```python
from build123d import *

# Parameters (mm, degrees)
SKETCH1_R      = 2.6035
EXTRUDE1_DEPTH = 25.4


with BuildPart() as part:
    # Sketch1 → Extrude1 (new body)
    with BuildSketch(Plane.XY):
        with BuildLine():
            Line((10.5918, 12.7), (10.5664, 12.7))
            ThreePointArc((10.5664, 12.7), (10.0584, 12.192), (9.5504, 12.7))
            Line((9.5504, 12.7), (6.3246, 12.7))
            ThreePointArc((6.3246, 12.7), (5.8166, 12.192), (5.3086, 12.7))
            Line((5.3086, 12.7), (4.3561, 12.7))
            ThreePointArc((4.3561, 12.7), (3.2512, 11.5951), (4.3561, 10.4902))
            Line((4.3561, 10.4902), (6.370083786, 10.4902))
            ThreePointArc((6.370083786, 10.4902), (7.348856743, 9.836204819), (7.119204175, 8.681663397))
            Line((7.119204175, 8.681663397), (3.88464389, 5.447103113))
            ThreePointArc((3.88464389, 5.447103113), (2.854599758, 4.758849627), (1.63957986, 4.517167143))
            Line((1.63957986, 4.517167143), (-1.63957986, 4.517167143))
            ThreePointArc((-1.63957986, 4.517167143), (-2.854599758, 4.758849627), (-3.88464389, 5.447103113))
            Line((-3.88464389, 5.447103113), (-7.119204175, 8.681663397))
            ThreePointArc((-7.119204175, 8.681663397), (-7.348856743, 9.836204819), (-6.370083786, 10.4902))
            Line((-6.370083786, 10.4902), (-4.3561, 10.4902))
            ThreePointArc((-4.3561, 10.4902), (-3.2512, 11.5951), (-4.3561, 12.7))
            Line((-4.3561, 12.7), (-5.3086, 12.7))
            ThreePointArc((-5.3086, 12.7), (-5.8166, 12.192), (-6.3246, 12.7))
            Line((-6.3246, 12.7), (-9.5504, 12.7))
            ThreePointArc((-9.5504, 12.7), (-10.0584, 12.192), (-10.5664, 12.7))
            Line((-10.5664, 12.7), (-10.5918, 12.7))
            ThreePointArc((-10.5918, 12.7), (-12.082522516, 12.082522516), (-12.7, 10.5918))
            Line((-12.7, 10.5918), (-12.7, 10.5664))
            ThreePointArc((-12.7, 10.5664), (-12.192, 10.0584), (-12.7, 9.5504))
            Line((-12.7, 9.5504), (-12.7, 6.3246))
            ThreePointArc((-12.7, 6.3246), (-12.192, 5.8166), (-12.7, 5.3086))
            Line((-12.7, 5.3086), (-12.7, 4.3561))
            ThreePointArc((-12.7, 4.3561), (-11.5951, 3.2512), (-10.4902, 4.3561))
            Line((-10.4902, 4.3561), (-10.4902, 6.370083786))
            ThreePointArc((-10.4902, 6.370083786), (-9.836204819, 7.348856743), (-8.681663397, 7.119204175))
            Line((-8.681663397, 7.119204175), (-5.447103113, 3.88464389))
            ThreePointArc((-5.447103113, 3.88464389), (-4.758849627, 2.854599758), (-4.517167143, 1.63957986))
            Line((-4.517167143, 1.63957986), (-4.517167143, -1.63957986))
            ThreePointArc((-4.517167143, -1.63957986), (-4.758849627, -2.854599758), (-5.447103113, -3.88464389))
            Line((-5.447103113, -3.88464389), (-8.681663397, -7.119204175))
            ThreePointArc((-8.681663397, -7.119204175), (-9.836204819, -7.348856743), (-10.4902, -6.370083786))
            Line((-10.4902, -6.370083786), (-10.4902, -4.3561))
            ThreePointArc((-10.4902, -4.3561), (-11.5951, -3.2512), (-12.7, -4.3561))
            Line((-12.7, -4.3561), (-12.7, -5.3086))
            ThreePointArc((-12.7, -5.3086), (-12.192, -5.8166), (-12.7, -6.3246))
            Line((-12.7, -6.3246), (-12.7, -9.5504))
            ThreePointArc((-12.7, -9.5504), (-12.192, -10.0584), (-12.7, -10.5664))
            Line((-12.7, -10.5664), (-12.7, -10.5918))
            ThreePointArc((-12.7, -10.5918), (-12.082522516, -12.082522516), (-10.5918, -12.7))
            Line((-10.5918, -12.7), (-10.5664, -12.7))
            ThreePointArc((-10.5664, -12.7), (-10.0584, -12.192), (-9.5504, -12.7))
            Line((-9.5504, -12.7), (-6.3246, -12.7))
            ThreePointArc((-6.3246, -12.7), (-5.8166, -12.192), (-5.3086, -12.7))
            Line((-5.3086, -12.7), (-4.3561, -12.7))
            ThreePointArc((-4.3561, -12.7), (-3.2512, -11.5951), (-4.3561, -10.4902))
            Line((-4.3561, -10.4902), (-6.370083786, -10.4902))
            ThreePointArc((-6.370083786, -10.4902), (-7.348856743, -9.836204819), (-7.119204175, -8.681663397))
            Line((-7.119204175, -8.681663397), (-3.88464389, -5.447103113))
            ThreePointArc((-3.88464389, -5.447103113), (-2.854599758, -4.758849627), (-1.63957986, -4.517167143))
            Line((-1.63957986, -4.517167143), (1.63957986, -4.517167143))
            ThreePointArc((1.63957986, -4.517167143), (2.854599758, -4.758849627), (3.88464389, -5.447103113))
            Line((3.88464389, -5.447103113), (7.119204175, -8.681663397))
            ThreePointArc((7.119204175, -8.681663397), (7.348856743, -9.836204819), (6.370083786, -10.4902))
            Line((6.370083786, -10.4902), (4.3561, -10.4902))
            ThreePointArc((4.3561, -10.4902), (3.2512, -11.5951), (4.3561, -12.7))
            Line((4.3561, -12.7), (5.3086, -12.7))
            ThreePointArc((5.3086, -12.7), (5.8166, -12.192), (6.3246, -12.7))
            Line((6.3246, -12.7), (9.5504, -12.7))
            ThreePointArc((9.5504, -12.7), (10.0584, -12.192), (10.5664, -12.7))
            Line((10.5664, -12.7), (10.5918, -12.7))
            ThreePointArc((10.5918, -12.7), (12.082522516, -12.082522516), (12.7, -10.5918))
            Line((12.7, -10.5918), (12.7, -10.5664))
            ThreePointArc((12.7, -10.5664), (12.192, -10.0584), (12.7, -9.5504))
            Line((12.7, -9.5504), (12.7, -6.3246))
            ThreePointArc((12.7, -6.3246), (12.192, -5.8166), (12.7, -5.3086))
            Line((12.7, -5.3086), (12.7, -4.3561))
            ThreePointArc((12.7, -4.3561), (11.5951, -3.2512), (10.4902, -4.3561))
            Line((10.4902, -4.3561), (10.4902, -6.370083786))
            ThreePointArc((10.4902, -6.370083786), (9.836204819, -7.348856743), (8.681663397, -7.119204175))
            Line((8.681663397, -7.119204175), (5.447103113, -3.88464389))
            ThreePointArc((5.447103113, -3.88464389), (4.758849627, -2.854599758), (4.517167143, -1.63957986))
            Line((4.517167143, -1.63957986), (4.517167143, 1.63957986))
            ThreePointArc((4.517167143, 1.63957986), (4.758849627, 2.854599758), (5.447103113, 3.88464389))
            Line((5.447103113, 3.88464389), (8.681663397, 7.119204175))
            ThreePointArc((8.681663397, 7.119204175), (9.836204819, 7.348856743), (10.4902, 6.370083786))
            Line((10.4902, 6.370083786), (10.4902, 4.3561))
            ThreePointArc((10.4902, 4.3561), (11.5951, 3.2512), (12.7, 4.3561))
            Line((12.7, 4.3561), (12.7, 5.3086))
            ThreePointArc((12.7, 5.3086), (12.192, 5.8166), (12.7, 6.3246))
            Line((12.7, 6.3246), (12.7, 9.5504))
            ThreePointArc((12.7, 9.5504), (12.192, 10.0584), (12.7, 10.5664))
            Line((12.7, 10.5664), (12.7, 10.5918))
            ThreePointArc((12.7, 10.5918), (12.082522516, 12.082522516), (10.5918, 12.7))
        make_face()
        Circle(SKETCH1_R, mode=Mode.SUBTRACT)
    extrude(amount=-EXTRUDE1_DEPTH)


solid = part.part
```
Geometry: final body of the model. Coordinates: model frame, mm. A direction names the side the tool comes from. Give positions to 0.01 mm unless a question says otherwise; leave off trailing zeros. Write each loop counter-clockwise with the first axis right and the second up, starting at its lowest first coordinate (ties: lowest second). Pieces come first, ordered by that corner, then holes.
1. Reachability of faces 4 (the cylindrical face through (12.192, 10.047, -12.522)), 5 (the cylindrical face through (11.57, 3.25, -12.52)), 6 (the flat face through (-4.517, 0, -13)) from +Z, -Z, +X, -X, +Y, -Y: full face, straight path, thin tool, end or side. Return the list, or none.
2. Section query A-A, the plane y = 0. Return loops of the section in (x, z), then the cut area to 3 significant figures.
3. Draft query along X for faces 1 (the flat face through (-12.7, 5, -13)), 2 (the cylindrical face through (-4.766, 2.871, -12.522)), 3 (the cylindrical face through (12.192, 5.805, -12.522)). Return one class per face: released by +X, released by -X, zero draft, split by the parting line, or undercut.
4. Line query: probe 1 along X at (y, z) = (-6.5, -16); probe 2 along X at (y, z) = (3.75, -9.5); probe 3 along Y at (x, z) = (0, -16.25). Output: solid intervals per line, ascending.
5. Pin query (flat end, axial travel): P1, Ø1, axis at y = 1.5, z = -13.5, coming from the +X side; P2, Ø1, axis at y = 0, z = -7.5, coming from the -X side; P3, Ø2, axis at x = -7.5, y = 1.5, coming from the -Z side; P4, Ø2.5, axis at x = 0, z = -11, coming from the +Y side. Return the tip coordinate at first contact, or that it passes through.
Computed:
1. face 4: +Z, -Z, +X
1. face 5: +Z, -Z
1. face 6: +Z, -Z, -X
2. outline: (-4.52, -25.4) - (-2.6, -25.4) - (-2.6, 0) - (-4.52, 0) - close; (2.6, -25.4) - (4.52, -25.4) - (4.52, 0) - (2.6, 0) - close
2. area: 97.2 mm2
3. face 1: released by -X
3. face 2: undercut
3. face 3: released by +X
4. probe 1: x = -12.7 to -10.48, -8.06 to -4.94, 4.94 to 8.06, 10.48 to 12.7
4. probe 2: x = -12.52 to -10.67, -5.32 to 5.32, 10.67 to 12.52
4. probe 3: y = -4.52 to -2.6, 2.6 to 4.52
5. P1: stops at x = 4.54
5. P2: stops at x = -4.52
5. P3: passes through
5. P4: stops at y = 4.52
